```python
from build123d import *

# Parameters (mm, degrees)
BOSS_EXTRUDE1_DEPTH = 3.175
SKETCH3_R           = 1.47
CUT_EXTRUDE5_DEPTH  = 10
CUT_EXTRUDE6_DEPTH  = 10


with BuildPart() as part:
    # Sketch1 → Boss-Extrude1 (new body)
    with BuildSketch(Plane.XY):
        Polygon((-26.794919243, 100), (26.794919243, 100), (73.205080757, 73.205080757), (100, 26.794919243), (100, -26.794919243), (73.205080757, -73.205080757), (26.794919243, -100), (-26.794919243, -100), (-73.205080757, -73.205080757), (-100, -26.794919243), (-100, 26.794919243), (-73.205080757, 73.205080757), align=None)
    extrude(amount=BOSS_EXTRUDE1_DEPTH)

    # Sketch3 → Cut-Extrude5 (cut)
    with BuildSketch(Plane(origin=(0, 0, 0), x_dir=(-1, 0, 0), z_dir=(0, 0, -1))):
        Polygon((51.443588913, -82.102909721), (53.031088913, -84.852540378), (73.205080757, -73.205080757), (84.852540378, -53.031088913), (82.102909721, -51.443588913), (70.880819443, -70.880819443), align=None)
        Polygon((-26.794919243, -100), (-3.5, -100), (-3.5, -96.825), (-25.944180557, -96.825), (-45.381411087, -85.602909721), (-46.968911087, -88.352540378), align=None)
        Polygon((-73.205080757, -73.205080757), (-53.031088913, -84.852540378), (-51.443588913, -82.102909721), (-70.880819443, -70.880819443), (-82.102909721, -51.443588913), (-84.852540378, -53.031088913), align=None)
        with Locations((-49.20625, -85.22772505)):
            Circle(SKETCH3_R)
        Polygon((-100, -26.794919243), (-88.352540378, -46.968911087), (-85.602909721, -45.381411087), (-96.825, -25.944180557), (-96.825, -3.5), (-100, -3.5), align=None)
        Polygon((-100, 26.794919243), (-100, 3.5), (-96.825, 3.5), (-96.825, 25.944180557), (-85.602909721, 45.381411087), (-88.352540378, 46.968911087), align=None)
        Polygon((-26.794919243, 100), (-46.968911087, 88.352540378), (-45.381411087, 85.602909721), (-25.944180557, 96.825), (-3.5, 96.825), (-3.5, 100), align=None)
        Polygon((26.794919243, 100), (3.5, 100), (3.5, 96.825), (25.944180557, 96.825), (45.381411087, 85.602909721), (46.968911087, 88.352540378), align=None)
        Polygon((73.205080757, 73.205080757), (53.031088913, 84.852540378), (51.443588913, 82.102909721), (70.880819443, 70.880819443), (82.102909721, 51.443588913), (84.852540378, 53.031088913), align=None)
        with Locations((-85.22772505, 49.20625)):
            Circle(SKETCH3_R)
        with Locations((-49.20625, 85.22772505)):
            Circle(SKETCH3_R)
        with Locations((0, 98.4125)):
            Circle(SKETCH3_R)
        with Locations((49.20625, 85.22772505)):
            Circle(SKETCH3_R)
        with Locations((85.22772505, 49.20625)):
            Circle(SKETCH3_R)
        with Locations((98.4125, 0)):
            Circle(SKETCH3_R)
        Polygon((96.825, -3.5), (96.825, -25.944180557), (85.602909721, -45.381411087), (88.352540378, -46.968911087), (100, -26.794919243), (100, -3.5), align=None)
        with Locations((85.22772505, -49.20625)):
            Circle(SKETCH3_R)
        Polygon((45.381411087, -85.602909721), (25.944180557, -96.825), (3.5, -96.825), (3.5, -100), (26.794919243, -100), (46.968911087, -88.352540378), align=None)
        with Locations((0, -98.4125)):
            Circle(SKETCH3_R)
        with Locations((49.20625, -85.22772505)):
            Circle(SKETCH3_R)
        with Locations((-85.22772505, -49.20625)):
            Circle(SKETCH3_R)
        with Locations((-98.4125, 0)):
            Circle(SKETCH3_R)
        Polygon((-82.102909721, 51.443588913), (-70.880819443, 70.880819443), (-51.443588913, 82.102909721), (-53.031088913, 84.852540378), (-73.205080757, 73.205080757), (-84.852540378, 53.031088913), align=None)
        Polygon((100, 26.794919243), (88.352540378, 46.968911087), (85.602909721, 45.381411087), (96.825, 25.944180557), (96.825, 3.5), (100, 3.5), align=None)
    extrude(amount=-CUT_EXTRUDE5_DEPTH, mode=Mode.SUBTRACT)

    # Sketch4 → Cut-Extrude6 (cut)
    with BuildSketch(Plane.XY.offset(3.175)):
        Polygon((27.531680557, 99.574630657), (25.944180557, 96.825), (96.825, -25.944180557), (101.705845195, -25.944180557), (99.574630657, 27.531680557), (73.205080757, 73.205080757), align=None)
    extrude(amount=-CUT_EXTRUDE6_DEPTH, mode=Mode.SUBTRACT)


solid = part.part
```
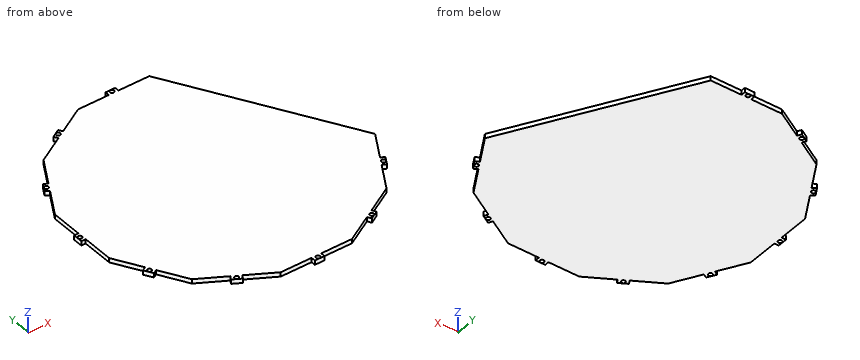
Check sheet for the modelled part. Datum: model origin and axes. Units: mm. Round coordinates to 2 decimals unless told otherwise and drop trailing zeros. Order: outer loops, then holes, each group sorted by start corner. A loop starts at its lowest first (then second) coordinate and runs counter-clockwise, first axis right, second up.
1) Section check A-A (x = 23.5). Record the boundary of the cut face in (y, z) (3 decimals).
2) Section check C-C (y = -20). Record the boundary of the cut face in (x, z) (3 decimals), and give its area (3 significant figures).
3) Section check B-B (z = 1.85). Give the number of separate pieces and of enclosed holes in the cut face, and give its area (3 significant figures).
4) Scan lines: line 1 (Y direction, x = -85.5, z = 0.8); line 2 (Y direction, x = -1, z = 1.85); line 3 (X direction, y = -88, z = 1.25). Record each from-to range of solid material in increasing order.
5) Go/stop test with flat-tipped pins: pin 1 Ø8 at (x, y) = (45.5, -68.5) entering from -Z; pin 2 Ø1.6 at (y, z) = (-97.5, 1.5) entering from +X; pin 3 Ø1 at (x, z) = (-17, 1) entering from -Y (3 decimals); pin 4 Ø1 at (y, z) = (-10.5, 1) entering from -X (3 decimals). Record where each tip stops, or that it passes through.
Result:
1. outline: (-96.825, 0) - (96.825, 0) - (96.825, 3.175) - (-96.825, 3.175) - close
2. outline: (-96.825, 0) - (93.393, 0) - (93.393, 3.175) - (-96.825, 3.175) - close
2. area: 604 mm2
3. separate pieces: 1
3. enclosed holes: 9
3. area: 27,800 mm2
4. line 1: y = -51.91 to -50.65, -47.76 to 47.76, 50.65 to 51.91
4. line 2: y = -100 to -99.49, -97.34 to 97.34, 99.49 to 100
4. line 3: x = -47.58 to -46.77, -41.23 to 41.23, 46.77 to 47.58
5. pin 1: stops at z = 0
5. pin 2: stops at x = 26.16
5. pin 3: stops at y = -96.825
5. pin 4: stops at x = -96.825
